from build123d import *

# Parameters (mm, degrees)
ESBO_O1_W                     = 70
ESBO_O1_H                     = 10
RESSALTO_EXTRUS_O1_DEPTH      = 1
RESSALTO_EXTRUS_O1_DEPTH_BACK = 2


with BuildPart() as part:
    # Esboço1 → Ressalto-extrusão1 (new body, two sides)
    with BuildSketch(Plane.XY) as ressalto_extrus_o1_sk:
        Polygon((-68.286430173, 37.282901017), (-120.286430173, 37.282901017), (-120.286430173, -27.717098983), (23.713569827, -27.717098983), (23.713569827, 37.282901017), (-28.286430173, 37.282901017), (-28.286430173, 34.282901017), (-68.286430173, 34.282901017), align=None)
        with Locations((-41.286430173, -7.717098983)):
            Rectangle(ESBO_O1_W, ESBO_O1_H, mode=Mode.SUBTRACT)
    extrude(amount=RESSALTO_EXTRUS_O1_DEPTH)
    extrude(ressalto_extrus_o1_sk.sketch, amount=-RESSALTO_EXTRUS_O1_DEPTH_BACK)


solid = part.part
The listing builds one solid part. Answer for the finished solid, in the listing's coordinates (mm). A direction names the side the tool comes from. Round coordinates to 2 decimals unless told otherwise and drop trailing zeros. Loops run counter-clockwise (first coordinate to the right, second up) from the corner with the lowest first, then second, coordinate; pieces in that order, holes last. Notation, with made-up numbers: M 72,1 L 115,1 A35 cw 115,34 Z; hole C 14,21 d2. An arc over 180 degrees is marked long. Write each question's results on one line, items separated by ' | '. Start each with the question number.
1) Find section A-A on x = -33.5. Write down the section's boundary in (y, z).
2) Determine the mould class of faces 1 (the flat face through (-68.286, 36, 0)), 2 (the flat face through (-120.286, 5, 0)), 3 (the flat face through (-94, 37.283, 0)) for opening direction X: pulls with the +X half, pulls with the -X half, needs draft (parallel to the pull), parting line crosses it, or undercut.
3) Which of the six approach directions +Z, -Z, +X, -X, +Y, -Y give full straight-line access (tool end or side, diameter ignored) to faces 4 (the flat face through (-6.286, -8, 0)), 5 (the flat face through (23.714, 4, 0)), 6 (the flat face through (-48, 34.283, 0))?
4) This flat-tipped pin is pushed along its axis until it touches: pin 1 (1.5 mm diameter, centred on x = -30, z = -1, fed in from +Y). Where does it stop, or does it pass through?
5) Find section B-B on y = -8. Write down the section's boundary in (x, z).
6) Find section C-C on z = -0.7. Write down the section's boundary in (x, y).
7) Straight lines are drawn through the part: probe 1 along Y at (x, z) = (-13, 0.4); probe 2 along X at (y, z) = (-10, -1.7); probe 3 along Y at (x, z) = (-39, -1.2). For each, find the intervals that lie inside material, in ascending order.
Final values:
1) outline: M -27.72,-2 L -12.72,-2 L -12.72,1 L -27.72,1 Z; M -2.72,-2 L 34.28,-2 L 34.28,1 L -2.72,1 Z
2) face 1: undercut | face 2: pulls with the -X half | face 3: needs draft
3) face 4: +Z, -Z | face 5: +Z, -Z, +X, +Y, -Y | face 6: +Z, -Z, +Y
4) pin 1: y = 34.28
5) outline: M -120.29,-2 L -76.29,-2 L -76.29,1 L -120.29,1 Z; M -6.29,-2 L 23.71,-2 L 23.71,1 L -6.29,1 Z
6) outline: M -120.29,-27.72 L 23.71,-27.72 L 23.71,37.28 L -28.29,37.28 L -28.29,34.28 L -68.29,34.28 L -68.29,37.28 L -120.29,37.28 Z; hole M -76.29,-12.72 L -6.29,-12.72 L -6.29,-2.72 L -76.29,-2.72 Z
7) probe 1: -27.72 to -12.72, -2.72 to 37.28 | probe 2: -120.29 to -76.29, -6.29 to 23.71 | probe 3: -27.72 to -12.72, -2.72 to 34.28
